Autodesk Inventor part; units mm, degrees
ref_plane "YZ Plane" through (0, 0, 0) normal (1, 0, 0) x (0, 1, 0)
ref_plane "XZ Plane" through (0, 0, 0) normal (0, 1, 0) x (-1, 0, 0)
ref_plane "XY Plane" through (0, 0, 0) normal (0, 0, 1) x (1, 0, 0)
sketch "Skizze1" plane through (0, 0, 0) normal (0, 0, 1) x (1, 0, 0)
  line L0 (-23.874, 0) -> (23.874, 0)
  line L1 (0, -27.4815) -> (0, 27.4815)
  line L2 (-16.9467, 9.9068) -> (0.1062, 19.6296)
  line L3 (0.1062, 19.6296) -> (17.0529, 9.7228)
  line L4 (17.0529, 9.7228) -> (16.9467, -9.9068)
  line L5 (16.9467, -9.9068) -> (-0.1062, -19.6296)
  line L6 (-0.1062, -19.6296) -> (-17.0529, -9.7228)
  line L7 (-17.0529, -9.7228) -> (-16.9467, 9.9068)
  circle A0 centre (0, 0) radius 15
  dimension "d0" = 30
  dimension "d1" = 17
extrude "Extrusion1" add sketch "Skizze1" along normal blind 20
sketch "Skizze3" plane through (0, 0, 20) normal (0, 0, 1) x (1, 0, 0)
  point P0 (0, 0)
hole "Bohrung1" at (0, 0, 20) direction (0, 0, -1) diameter 26.211 depth 18
chamfer "Fase1" distance 0.5 angle 45 1 edges at (0, 13.1055, 20)
properties part number "VerteilerLuft2"
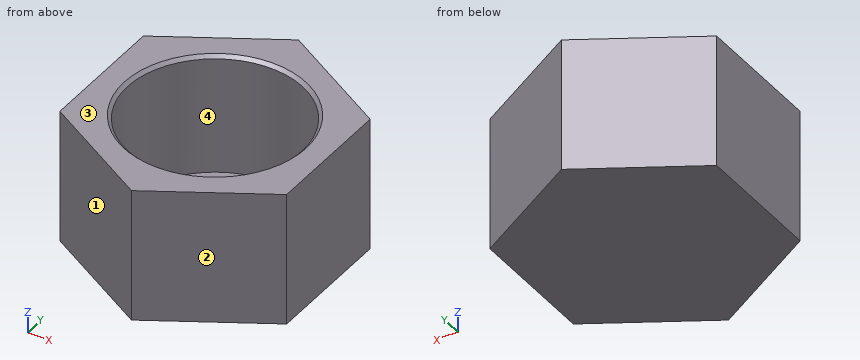
Verification items for the finished model (mm, model axes). Face numbers are marked on the shaded views. Give positions to 0.01 mm unless a question says otherwise; leave off trailing zeros. Loops run counter-clockwise (first coordinate to the right, second up) from the corner with the lowest first, then second, coordinate; pieces in that order, holes last.
1. Section check D-D, the plane y = -15. Enter the section's corners in (x, z), then the cut area to 3 significant figures.
2. Section check C-C, the plane x = 15. Enter the section's corners in (y, z).
3. Go/stop test with flat-tipped pins: pin 1 Ø4 at (y, z) = (14, 9.5) entering from +X; pin 2 Ø1 at (y, z) = (5, 12.5) entering from -X; pin 3 Ø10 at (x, z) = (-6.5, 9) entering from +Y; pin 4 Ø2 at (x, y) = (-9, 14.5) entering from +Z. Record where each tip stops, or that it passes through.
4. Section check A-A, the plane z = 17. Enter the section's corners in (x, y), then the cut area to 3 significant figures.
5. Thickness scan on line 1 (X direction, y = -4.5, z = 10.75); line 2 (Y direction, x = 9, z = 7.5); line 3 (X direction, y = 0, z = 10). Record the ranges inside material, lowest first.
6. Section check B-B, the plane y = 0. Enter the section's corners in (x, z), then the cut area to 3 significant figures.
7. Mould release check, pull along X, two halves, no side actions. Record for the marked faces 1, 2, 3 and 4: released by +X, released by -X, zero draft, split by the parting line, or undercut.
Geometry says:
1. outline: (-8.03, 0) - (8.01, 0) - (8.01, 20) - (-8.03, 20) - close
1. area: 321 mm2
2. outline: (-11.02, 0) - (10.92, 0) - (10.92, 20) - (-11.02, 20) - close
3. pin 1: stops at x = 13.16
3. pin 2: stops at x = -16.98
3. pin 3: stops at y = 18.71
3. pin 4: stops at z = 20
4. outline: (-17.05, -9.72) - (-0.11, -19.63) - (16.95, -9.91) - (17.05, 9.72) - (0.11, 19.63) - (-16.95, 9.91) - close; hole circle Ø26.21 at (0, 0)
4. area: 462 mm2
5. line 1: x = -17.02 to -12.31, 12.31 to 16.98
5. line 2: y = -14.44 to -9.53, 9.53 to 14.43
5. line 3: x = -17 to -13.11, 13.11 to 17
6. outline: (-17, 0) - (17, 0) - (17, 20) - (13.61, 20) - (13.11, 19.5) - (13.11, 2) - (-13.11, 2) - (-13.11, 19.5) - (-13.61, 20) - (-17, 20) - close
6. area: 208 mm2
7. face 1: released by -X
7. face 2: released by +X
7. face 3: zero draft
7. face 4: undercut
